Input: part model. Units: mm. Frame: model coordinates. A direction names the side the tool comes from. Give positions to 0.01 mm unless a question says otherwise; leave off trailing zeros. Loops run counter-clockwise (first coordinate to the right, second up) from the corner with the lowest first, then second, coordinate; pieces in that order, holes last. Notation, with made-up numbers: (-11, -14) - (5, -14) arc R19 ccw to (5, 8) - close; hole circle Ø2 at (3, 67.25). An arc over 180 degrees is marked (long way). Answer as a JSON object with one key per item and string values. Group by question number.
(1) Section query A-A (z = -16). Return loops of the section in (x, y), plus the area to 3 significant figures.
(2) Section query B-B (z = -23.25). Return loops of the section in (x, y).
(3) Access query for faces 4 (the flat face through (-3.916, -6.638, -12.177)), 5 (the flat face through (8, 14, -24.7)). Directions: +Z, -Z, +X, -X, +Y, -Y. A direction counts if a zero-diameter tool reaches every point of the face in a straight line with its end or side. Return the directions, or none.
(4) Mould query, pull axis X, two halves, no side actions, for faces 1 (the flat face through (3, -7, -24.7)), 2 (the cylindrical face through (10.735, 2.602, -0.386)), 3 (the cylindrical face through (5.841, -7.869, -8.154)). Classes: +X half, -X half, draft (parallel to the pull), parting line (faces both ways), or undercut.
(5) Pin query (flat end, axial travel): P1, Ø12, axis at x = 12.5, z = -9, coming from the +Y side; P2, Ø6, axis at x = 6, y = -7, coming from the -Z side; P3, Ø5, axis at x = -1.5, z = -9, coming from the +Y side. Return the tip coordinate at first contact, or that it passes through.
(6) Material intervals for L1, parallel to Y at x = 4.5, z = -14.75; L2, parallel to Y at x = 10.25, z = -15.5; L3, parallel to Y at x = -1, z = -3, sorted ascending.
```python
from build123d import *

# Parameters (mm, degrees)
RESSALTO_EXTRUS_O1_DEPTH = 25.5
CORTE_EXTRUS_O1_DEPTH    = 30.19013409
ESBO_O3_R                = 12
CORTE_EXTRUS_O2_DEPTH    = 22.755596158


with BuildPart() as part:
    # Esboço1 → Ressalto-extrusão1 (new body)
    with BuildSketch(Plane.XY):
        with BuildLine():
            Line((17.433095525, 13.814174971), (2.097319146, 17.616011747))
            Line((2.097319146, 17.616011747), (1.665269548, 15.873218352))
            ThreePointArc((1.665269548, 15.873218352), (10.676806339, 2.353151612), (-3.606507064, -5.391973191))
            Line((-3.606507064, -5.391973191), (-4.038556662, -7.134766585))
            Line((-4.038556662, -7.134766585), (11.297219716, -10.936603361))
            Line((11.297219716, -10.936603361), (17.433095525, 13.814174971))
        make_face()
    extrude(amount=-RESSALTO_EXTRUS_O1_DEPTH)

    # Esboço2 → Corte-extrusão1 (cut, through all)
    with BuildSketch(Plane(origin=(4.235701857, 17.085893034, 0), x_dir=(0, 0, 1), z_dir=(0.240622581, 0.970618758, 0))):
        Polygon((-24.7, -2.203112904), (-24.7, 8.696887096), (-25.5, 13.596887096), (-25.5, -2.203112904), align=None)
    extrude(amount=-CORTE_EXTRUS_O1_DEPTH, mode=Mode.SUBTRACT)

    # Esboço3 → Corte-extrusão2 (cut, through all)
    with BuildSketch(Plane(origin=(13.197393668, -3.271718063, 0), x_dir=(-0.240622581, -0.970618758, 0), z_dir=(0.970618758, -0.240622581, 0))):
        with Locations((-4.853093791, 12.75)):
            Circle(ESBO_O3_R)
    extrude(amount=-CORTE_EXTRUS_O2_DEPTH, mode=Mode.SUBTRACT)


solid = part.part
```
Recorded:
{
 "1": {"outline": "(-4.04, -7.13) - (11.3, -10.94) - (11.59, -9.77) - (-3.75, -5.97) - close; (1.81, 16.45) - (17.14, 12.65) - (17.43, 13.81) - (2.1, 17.62) - close", "area": "37.9 mm^2"},
 "2": {"outline": "(-4.04, -7.13) - (11.3, -10.94) - (12.97, -4.2) - (7.67, -2.89) arc R11 cw to (-3.61, -5.39) - close; (1.67, 15.87) arc R11 cw to (10.46, 8.39) - (15.76, 7.08) - (17.43, 13.81) - (2.1, 17.62) - close"},
 "3": {"face 4": "+Z, -Z, -X, +Y", "face 5": "-Z, -X, +Y"},
 "4": {"face 1": "draft", "face 2": "undercut", "face 3": "parting line"},
 "5": {"P1": "stops at y = 16.52", "P2": "stops at z = -25", "P3": "stops at y = -5.39"},
 "6": {"L1": "y = -9.25 to -8.31, 16.07 to 17.02", "L2": "y = -10.68 to -9.58, 14.49 to 15.59", "L3": "y = -7.89 to -5.95"}
}
